Read the model definition and answer for the solid it produces. Units are mm, in the model's axes. A direction names the side the tool comes from. Coordinates: 2 decimals unless noted, no trailing zeros. Write each loop counter-clockwise with the first axis right and the second up, starting at its lowest first coordinate (ties: lowest second). Pieces come first, ordered by that corner, then holes. Notation, with made-up numbers: (85.25, -0.5) -> (135.25, -0.5) arc R15 cw to (135.25, 12.5) -> close; hole circle Ø8 at (58, -9.75). An arc over 180 degrees is marked (long way). One line per item, written item: value. Start each with the question number.
1. Given P1, Ø19, axis at x = 0.5, y = 22, coming from the +Z side; P2, Ø1, axis at x = 4, y = 36.5, coming from the -Z side; P3, Ø4, axis at y = -44, z = 26, coming from the -X side; P4, Ø2, axis at x = 29, y = 44, coming from the +Z side, each flat-ended and moving along its own axis, determine where each tip first touches the part or whether it passes through.
2. Consider line 1 along Y through (x, z) = (17, -20); line 2 along Z through (x, y) = (-8.5, 13); line 3 along Y through (x, z) = (6, 0). Determine where each line is inside the solid, lowest interval first.
3. For a pull along Y with two mould halves and no side action, classify faces 6 (the flat face through (0.5, -52, -39.5)), 7 (the flat face through (-31, -42, -28)), 8 (the cylindrical face through (-21, -52, 28)) as pulls with the +Y half, pulls with the -Y half, needs draft (parallel to the pull), parting line crosses it, or undercut.
4. For faces 1 (the cylindrical face through (0.66, -60.93, 14.985)), 2 (the flat face through (-0.5, -52, 39.5)), 3 (the cylindrical face through (-19.642, 27.015, -0.66)), 4 (the cylindrical face through (-29.11, -20.49, 26.7)), 5 (the flat face through (33.8, -52, -20.5)), determine the directions among +Z, -Z, +X, -X, +Y, -Y from which every point of the face is accessible in a straight line to the end or side of a thin tool.
5. Find section A-A, the plane y = 12.5. Write down the section's boundary in (x, z).
6. Find section C-C, the plane y = 49.5. Write down the section's boundary in (x, z).
7. Find section B-B, the plane y = 29. Write down the section's boundary in (x, z), and give its area (3 significant figures).
```python
from build123d import *

# Parameters (mm, degrees)
SKETCH2_R            = 39.5
BOSS_EXTRUDE1_DEPTH  = 1
SKETCH4_R            = 41.25
BOSS_EXTRUDE2_DEPTH  = 1
SKETCH5_R            = 42
BOSS_EXTRUDE3_DEPTH  = 7
SKETCH6_R            = 35
BOSS_EXTRUDE4_DEPTH  = 7
BOSS_EXTRUDE7_DEPTH  = 3
CIRPATTERN2_COUNT    = 12
SKETCH8_R            = 15
BOSS_EXTRUDE8_DEPTH  = 10
SKETCH9_W            = 24
SKETCH9_H            = 40
BOSS_EXTRUDE9_DEPTH  = 42
BOSS_EXTRUDE10_START = -24
BOSS_EXTRUDE10_DEPTH = 24
SKETCH11_R           = 15
BOSS_EXTRUDE11_DEPTH = 15.5
BOSS_EXTRUDE12_START = 15.5
SKETCH12_R           = 15
BOSS_EXTRUDE12_DEPTH = 15.5


with BuildPart() as part:
    # Sketch1 → Revolve1 (revolve)
    with BuildSketch(Plane.XY):
        with BuildLine():
            Line((0, 0), (-35, 0))
            ThreePointArc((-35, 0), (-39.657515479, -9.46062113), (-40, -20))
            Line((-40, -20), (0, -20))
            Line((0, -20), (0, 0))
        make_face()
    revolve(axis=Axis((0, 0, 0), (0, -1, 0)))

    # Sketch2 → Boss-Extrude1 (add)
    with BuildSketch(Plane.XZ.offset(20)):
        Circle(SKETCH2_R)
    extrude(amount=BOSS_EXTRUDE1_DEPTH)

    # Sketch3 → Revolve2 (revolve)
    with BuildSketch(Plane(origin=(0, 0, 0), x_dir=(0, 0, -1), z_dir=(1, 0, 0)), mode=Mode.PRIVATE) as revolve2_sk:
        with BuildLine():
            Line((0, -21), (-40, -21))
            ThreePointArc((-40, -21), (-42.384109041, -30.861589096), (-42, -41))
            Line((-42, -41), (0, -41))
            Line((0, -41), (0, -21))
        make_face()
    revolve(revolve2_sk.sketch.rotate(Axis((0, -21, 0), (0, -1, 0)), 90), axis=Axis((0, -21, 0), (0, -1, 0)))

    # Sketch4 → Boss-Extrude2 (add)
    with BuildSketch(Plane.XZ.offset(41)):
        with Locations(Location((0, 0, 0), (0, 0, 270))):
            Circle(SKETCH4_R)
    extrude(amount=BOSS_EXTRUDE2_DEPTH)

    # Sketch5 → Boss-Extrude3 (add)
    with BuildSketch(Plane.XZ.offset(42)):
        with Locations(Location((0, 0, 0), (0, 0, 270))):
            Circle(SKETCH5_R)
    extrude(amount=BOSS_EXTRUDE3_DEPTH)

    # Sketch6 → Boss-Extrude4 (add)
    with BuildSketch(Plane.XZ.offset(49)):
        with Locations(Location((0, 0, 0), (0, 0, 270))):
            Circle(SKETCH6_R)
    extrude(amount=BOSS_EXTRUDE4_DEPTH)

    # Sketch7 → Boss-Extrude7 (add)
    with BuildSketch(Plane.XZ.offset(49)):
        Polygon((40.75, 0), (39.625, 1.948557159), (37.375, 1.948557159), (36.25, 0), (37.375, -1.948557159), (39.625, -1.948557159), align=None)
        Polygon((39.047649731, 0.948557159), (37.952350269, 0.948557159), (37.404700538, 0), (37.952350269, -0.948557159), (39.047649731, -0.948557159), (39.595299462, 0), align=None, mode=Mode.SUBTRACT)
    boss_extrude7 = extrude(amount=BOSS_EXTRUDE7_DEPTH)

    # CirPattern2: Boss-Extrude7 ×12 about axis
    cirpattern2_axis = Axis((0, 0, 0), (0, 1, 0))
    for i in range(1, CIRPATTERN2_COUNT):
        add(boss_extrude7.rotate(cirpattern2_axis, i * 360 / CIRPATTERN2_COUNT))

    # Sketch8 → Boss-Extrude8 (add)
    with BuildSketch(Plane.XZ.offset(56)):
        with Locations(Location((0, 0, 0), (0, 0, 270))):
            Circle(SKETCH8_R)
    extrude(amount=BOSS_EXTRUDE8_DEPTH)

    # Sketch9 → Boss-Extrude9 (add)
    with BuildSketch(Plane(origin=(0, 0, 0), x_dir=(1, 0, 0), z_dir=(0, 1, 0))):
        Rectangle(SKETCH9_W, SKETCH9_H)
    extrude(amount=BOSS_EXTRUDE9_DEPTH)

    # Sketch10 → Boss-Extrude10 (add)
    with BuildSketch(Plane.ZY.offset(12).offset(BOSS_EXTRUDE10_START)):
        with BuildLine():
            Line((-20, 42), (20, 42))
            ThreePointArc((20, 42), (0, 62), (-20, 42))
        make_face()
    extrude(amount=BOSS_EXTRUDE10_DEPTH)

    # Sketch11 → Boss-Extrude11 (add)
    with BuildSketch(Plane.ZY.offset(12)):
        with Locations(Location((0, 42, 0), (0, 0, 90))):
            Circle(SKETCH11_R)
    extrude(amount=BOSS_EXTRUDE11_DEPTH)

    # Sketch12 → Boss-Extrude12 (add)
    with BuildSketch(Plane(origin=(12, 0, 0), x_dir=(0, 0, -1), z_dir=(1, 0, 0)).offset(BOSS_EXTRUDE12_START)):
        with Locations(Location((0, 42, 0), (0, 0, 90))):
            Circle(SKETCH12_R)
    extrude(amount=-BOSS_EXTRUDE12_DEPTH)


solid = part.part
```
Answer block:
1. P1: stops at z = 20
1. P2: stops at z = -20
1. P3: stops at x = -34.47
1. P4: passes through
2. line 1: y = -56 to 0
2. line 2: z = -20 to 20
2. line 3: y = -66 to 62
3. face 6: pulls with the -Y half
3. face 7: undercut
3. face 8: needs draft
4. face 1: -Y
4. face 2: +Z, +X, -X, -Y
4. face 3: -X
4. face 4: none
4. face 5: -Z, +X, -Y
5. outline: (-12, -20) -> (12, -20) -> (12, 20) -> (-12, 20) -> close
6. outline: (-27.5, -12.99) -> (-12, -12.99) -> (-12, -18.54) -> (12, -18.54) -> (12, -12.99) -> (27.5, -12.99) -> (27.5, 12.99) -> (12, 12.99) -> (12, 18.54) -> (-12, 18.54) -> (-12, 12.99) -> (-27.5, 12.99) -> close
7. outline: (-27.5, -7.48) -> (-12, -7.48) -> (-12, -20) -> (12, -20) -> (12, -7.48) -> (27.5, -7.48) -> (27.5, 7.48) -> (12, 7.48) -> (12, 20) -> (-12, 20) -> (-12, 7.48) -> (-27.5, 7.48) -> close
7. area: 1,420 mm2
